Source: CAD feature listing. Evaluate the final solid. Frame: model axes, mm. A direction names the side the tool comes from. Round coordinates to 2 decimals unless told otherwise and drop trailing zeros. Order: outer loops, then holes, each group sorted by start corner. A loop starts at its lowest first (then second) coordinate and runs counter-clockwise, first axis right, second up. Notation, with made-up numbers: (23.25, 76) - (32.25, 76) arc R20 ccw to (32.25, 83) - close; hole circle Ø3 at (23, 12.25). An arc over 180 degrees is marked (long way). Put each result on its own line as item: value. Start each with the question number.
1) Section C-C on x = -8. Output: boundary loops of the cut face in (y, z), then the cut area to 3 significant figures.
2) Section A-A on y = 8. Output: boundary loops of the cut face in (x, z).
3) Section D-D on y = 13. Output: boundary loops of the cut face in (x, z) (3 decimals), then the cut area to 3 significant figures.
4) Access query for faces 1 (the face through (-3, 8.1, -13.6)), 2 (the face through (-1.521, 1.428, -18.645)). Directions: +Z, -Z, +X, -X, +Y, -Y. A direction counts if a zero-diameter tool reaches every point of the face in a straight line with its end or side. Return the directions, or none.
5) Mould query, pull axis X, two halves, no side actions, for faces 3 (the face through (0, 8, -12)), 4 (the face through (-16, 8, -12)), 5 (the face through (-8, 8, -7)), 6 (the face through (-15, 8, -20)). Classes: +X half, -X half, draft (parallel to the pull), parting line (faces both ways), or undercut.
6) Contact query for a flat-ended pin moving along its axis: P1, Ø2.5, axis at x = -8, y = 3, coming from the -Z side. Output: stop coordinate, or through.
7) Section B-B on z = -16.25. Output: boundary loops of the cut face in (x, y), then the cut area to 3 significant figures.
8) Line query: probe 1 along Z at (x, y) = (-2.2, 8); probe 2 along X at (y, z) = (4.25, -14); probe 3 along Y at (x, z) = (-2.4, -15). Output: solid intervals per line, ascending. Write a range as [from, to].
Autodesk Inventor part; units mm, degrees
ref_plane "Work Plane1" through (0, 0, -15) normal (0, 0, -1) x (-1, 0, 0)
ref_plane "YZ Plane" through (0, 0, 0) normal (1, 0, 0) x (0, 1, 0)
ref_plane "XZ Plane" through (0, 0, 0) normal (0, 1, 0) x (-1, 0, 0)
sketch "Sketch1" plane through (0, 0, 0) normal (0, 1, 0) x (-1, 0, 0)
  line L0 (0, 0) -> (16, 0)
  line L1 (16, 0) -> (16, -20)
  line L2 (16, -20) -> (0, -20)
  line L3 (0, -20) -> (0, 0)
  dimension "d0" = 16
  dimension "d1" = 20
extrude "Extrusion1" add sketch "Sketch1" along normal blind 16
ref_plane "Work Plane1" through (0, 0, -15) normal (0, 0, -1) x (-1, 0, 0)
sketch "Sketch2" plane through (0, 0, -15) normal (0, 0, -1) x (-1, 0, 0)
  line L0 (16, 16) -> (0, 16)
  line L1 (8, 16) -> (3, 16)
  line L2 (3, 16) -> (13, 16)
  line L3 (0, 0) -> (0, 16)
  line L4 (0, 8) -> (3, 8)
  line L5 (3, 8) -> (13, 8)
  line L6 (13, 8) -> (13, 16)
  line L7 (13, 16) -> (3, 16)
  line L8 (3, 16) -> (3, 8)
  dimension "d5" = 5
revolve "Revolution1" cut sketch "Sketch2" angle 360 about axis through (-3, 8, -15) along (-1, 0, 0) contours L6 L5 L8 L0
fillet "Fillet1" radius 4.75 4 edges at (-8, 14.245, -20) (-8, 1.755, -20) (-8, 16, -20) (-8, 0, -20)
sketch "Sketch3" plane through (-16, 0, 0) normal (0, 0, 1) x (1, 0, 0)
  line L0 (0, 16) -> (16, 16)
  line L1 (0, 16) -> (16, 16)
  line L2 (16, 16) -> (16, 0)
  line L3 (16, 0) -> (0, 0)
  line L4 (0, 0) -> (0, 16)
extrude "Extrusion2" cut sketch "Sketch3" against normal blind 4
sketch "Sketch4" plane through (0, 4.75, -20) normal (1, 0, 0) x (0, 0, -1)
  arc A0 (-5, 11.25) -> (-5, -4.75) centre (-5, 3.25) ccw
  circle A1 centre (-5, 3.25) radius 1
  point P0 (-20, -4.75)
  dimension "d12" = 2
extrude "Extrusion3" cut sketch "Sketch4" against normal up to surface (16 mm away)
sketch "Sketch5" plane through (-16, 0, -4) normal (0, 0, 1) x (1, 0, 0)
  line L0 (0, 16) -> (16, 16)
  circle A0 centre (8, 3) radius 1
  circle A1 centre (8, 13) radius 1
  point P0 (16, 0)
  dimension "d16" = 2
extrude "Extrusion4" cut sketch "Sketch5" against normal blind 10
sketch "Sketch6" plane through (0, 16, 0) normal (0, 1, 0) x (1, 0, 0)
  line L0 (-13, 15) -> (-3, 15)
  line L1 (-13, 16.0838) -> (-3, 16.0838)
  line L2 (-3, 15) -> (-13, 15)
  line L3 (-13, 15) -> (-13, 16.0838)
  line L4 (-13, 16.0838) -> (-3, 16.0838)
  line L5 (-3, 16.0838) -> (-3, 15)
  point P0 (0, 0)
extrude "Extrusion5" cut sketch "Sketch6" against normal up to surface (16 mm away)
properties part number "Bearing_Holder"
Answer sheet:
1. outline: (0, -15) arc R8 cw to (2, -9.71) - (2, -4) - (0, -4) - close; (4, -8.07) arc R8 cw to (12, -8.07) - (12, -4) - (4, -4) - close; (14, -9.71) arc R8 cw to (16, -15) - (16, -4) - (14, -4) - close
1. area: 56.3 mm^2
2. outline: (-16, -20) - (-13, -20) - (-13, -16) - (-16, -16) - close; (-16, -14) - (-13, -14) - (-13, -7) - (-3, -7) - (-3, -14) - (0, -14) - (0, -4) - (-16, -4) - close; (-3, -20) - (0, -20) - (0, -16) - (-3, -16) - close
3. outline: (-16, -19.666) - (-13, -19.666) - (-13, -8.755) - (-9, -8.755) - (-9, -4) - (-16, -4) - close; (-7, -8.755) - (-3, -8.755) - (-3, -19.666) - (0, -19.666) - (0, -4) - (-7, -4) - close
3. area: 132 mm^2
4. face 1: -Z
4. face 2: -Z, +X, -X, -Y
5. face 3: +X half
5. face 4: -X half
5. face 5: undercut
5. face 6: draft
6. P1: z = -10.01
7. outline: (-16, 0.11) - (-13, 0.11) - (-13, 15.89) - (-16, 15.89) - close; (-3, 0.11) - (0, 0.11) - (0, 15.89) - (-3, 15.89) - close
7. area: 94.7 mm^2
8. probe 1: [-20, -16], [-14, -4]
8. probe 2: [-16, -13], [-3, 0]
8. probe 3: [0, 7], [9, 16]
